Check sheet for the drawn part. Datum: minimum x, y, z corner. Units: mm. A direction names the side the tool comes from. Round coordinates to 2 decimals unless told otherwise and drop trailing zeros. Loops run counter-clockwise (first coordinate to the right, second up) from the corner with the lowest first, then second, coordinate; pieces in that order, holes last. Notation, with made-up numbers: (-17, 77) -> (5, 77) arc R22 cw to (5, 105) -> close; hole circle Ø3 at (63.5, 68). An arc over 180 degrees is marked (long way). Write item = value, one per line. Start each with the question number.
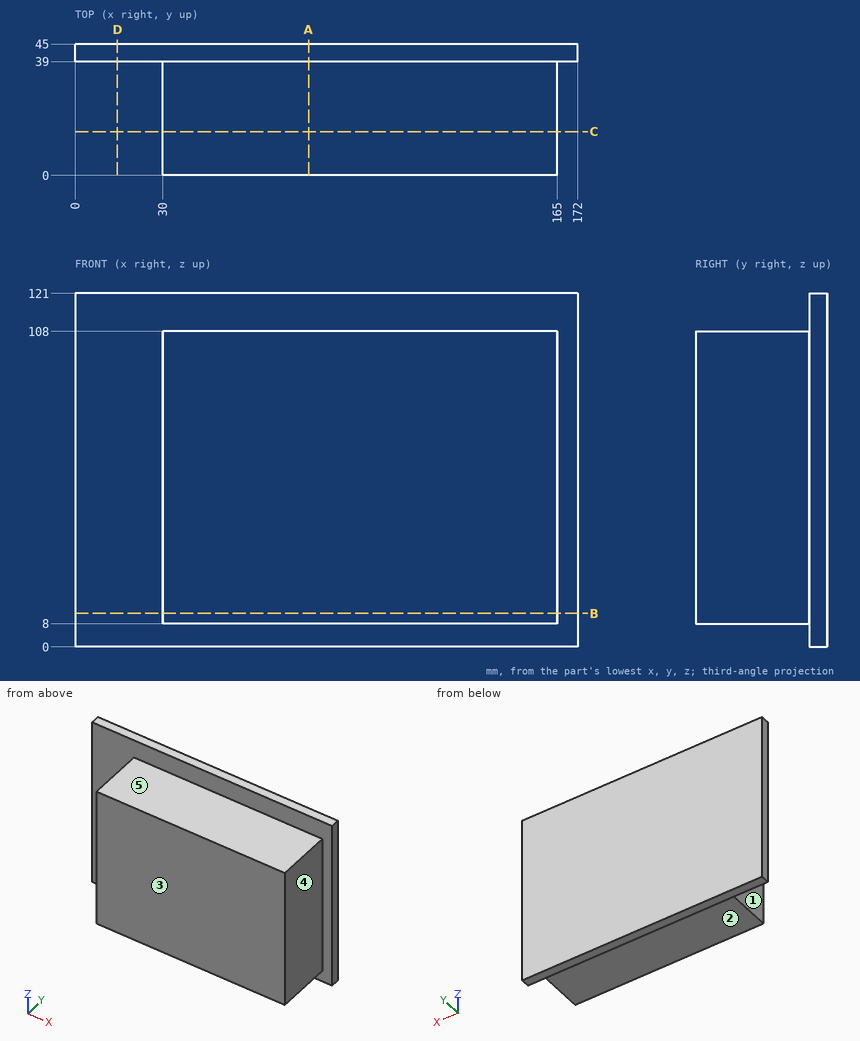
(1) Section check A-A on x = 80. Enter the section's corners in (y, z), then the cut area to 3 significant figures.
(2) Section check C-C on y = 15. Enter the section's corners in (x, z), then the cut area to 3 significant figures.
(3) Section check B-B on z = 11.5. Enter the section's corners in (x, y).
(4) Depth check by flat-ended pin: pin 1 Ø10 at (x, y) = (58, 32) entering from +Z; pin 2 Ø5 at (y, z) = (9.5, 19) entering from -X; pin 3 Ø3 at (x, y) = (59, 30.5) entering from -Z. Enter the tip coordinate at first touch or a pass-through.
(5) Access from +Z, -Z, +X, -X, +Y, -Y to the whole of each face (thin tool, end or side, straight path). Record for the marked faces 1, 2, 3, 4 and 5.
(6) Section check D-D on x = 14.5. Enter the section's corners in (y, z).
(7) Scan lines: line 1 (X direction, y = 33.5, z = 95); line 2 (Z direction, x = 129, y = 26); line 3 (Y direction, x = 158.5, z = 111.5). Record each from-to range of solid material in increasing order. Write a range as [from, to].
Computed values:
q1.outline = (0, 8) -> (39, 8) -> (39, 0) -> (45, 0) -> (45, 121) -> (39, 121) -> (39, 108) -> (0, 108) -> close
q1.area = 4,630 mm²
q2.outline = (30, 8) -> (165, 8) -> (165, 108) -> (30, 108) -> close
q2.area = 13,500 mm²
q3.outline = (0, 39) -> (30, 39) -> (30, 0) -> (165, 0) -> (165, 39) -> (172, 39) -> (172, 45) -> (0, 45) -> close
q4.pin_1 = 108
q4.pin_2 = 30
q4.pin_3 = 8
q5.face_1 = +Z, -Z, -X, -Y
q5.face_2 = -Z, +X, -X, -Y
q5.face_3 = +Z, -Z, +X, -X, -Y
q5.face_4 = +Z, -Z, +X, -Y
q5.face_5 = +Z, +X, -X, -Y
q6.outline = (39, 0) -> (45, 0) -> (45, 121) -> (39, 121) -> close
q7.line_1 = [30, 165]
q7.line_2 = [8, 108]
q7.line_3 = [39, 45]
